Source: CAD feature listing. Evaluate the final solid. Frame: model axes, mm. A direction names the side the tool comes from. Coordinates: 2 decimals unless noted, no trailing zeros. Loops run counter-clockwise (first coordinate to the right, second up) from the corner with the lowest first, then second, coordinate; pieces in that order, holes last.
Item 1: Section query A-A, the plane x = 26. Return the cut outline in (y, z).
Item 2: Reachability of faces 1 (the flat face through (28, 0, 0)), 2 (the flat face through (28, -0.26, 0)), 3 (the flat face through (36, 0.013, 0)) from +Z, -Z, +X, -X, +Y, -Y: full face, straight path, thin tool, end or side. Return the list, or none.
Item 3: Line query: probe 1 along X at (y, z) = (-0.05, -8.25); probe 2 along Y at (x, z) = (36, -1.75); probe 3 along Z at (x, y) = (65.5, -0.1). Output: solid intervals per line, ascending.
Item 4: Section query D-D, the plane x = 10.5. Return the cut outline in (y, z).
Item 5: Pin query (flat end, axial travel): pin 1 Ø4 at (x, z) = (35.5, -1.5) entering from +Y. Return the tip coordinate at first contact, or that it passes through.
Item 6: Section query B-B, the plane y = -0.1. Return the cut outline in (x, z), then the cut area to 4 significant figures.
```python
from build123d import *

# Parameters (mm, degrees)
BOSS_EXTRUDE1_DEPTH      = 0.0001
BOSS_EXTRUDE1_DEPTH_BACK = 0.26
BOSS_EXTRUDE2_DEPTH      = 0.0126
BOSS_EXTRUDE3_DEPTH      = 0.0666


with BuildPart() as part:
    # Sketch1 → Boss-Extrude1 (new, two sides: drawn at the far end of the back side and taken through both)
    with BuildSketch(Plane(origin=(0, 0, 0), x_dir=(1, 0, 0), z_dir=(0, 1, 0)).offset(-BOSS_EXTRUDE1_DEPTH_BACK)):
        Polygon((0, -15), (30, -15), (30, -5), (74.5, -5), (74.5, 5), (30, 5), (30, 15), (0, 15), align=None)
    extrude(amount=BOSS_EXTRUDE1_DEPTH + BOSS_EXTRUDE1_DEPTH_BACK)

    # Sketch3 → Boss-Extrude2 (add)
    with BuildSketch(Plane(origin=(0, 0.0001, 0), x_dir=(1, 0, 0), z_dir=(0, 1, 0))):
        Polygon((30, 3.75), (30, 1.25), (35.5, 1.25), (35.5, -1.25), (30, -1.25), (30, -3.75), (38, -3.75), (38, 3.75), align=None)
    extrude(amount=BOSS_EXTRUDE2_DEPTH)

    # Sketch4 → Boss-Extrude3 (add)
    with BuildSketch(Plane(origin=(0, 0.0001, 0), x_dir=(1, 0, 0), z_dir=(0, 1, 0))):
        Polygon((4, 10.25), (4, 1.25), (30, 1.25), (30, 3.75), (20.627589053, 3.75), (20.627589053, 10.25), align=None)
        Polygon((30, -1.25), (4, -1.25), (4, -10.25), (20.627589053, -10.25), (20.627589053, -3.75), (30, -3.75), align=None)
    extrude(amount=BOSS_EXTRUDE3_DEPTH)


solid = part.part
```
Verdict:
1. outline: (-0.26, -15) - (0, -15) - (0, -3.75) - (0.07, -3.75) - (0.07, -1.25) - (0, -1.25) - (0, 1.25) - (0.07, 1.25) - (0.07, 3.75) - (0, 3.75) - (0, 15) - (-0.26, 15) - close
2. face 1: +Y
2. face 2: +Z, -Z, +X, -X, -Y
2. face 3: +Z, -Z, +X, +Y
3. probe 1: x = 0 to 30
3. probe 2: y = -0.26 to 0.01
3. probe 3: z = -5 to 5
4. outline: (-0.26, -15) - (0, -15) - (0, -10.25) - (0.07, -10.25) - (0.07, -1.25) - (0, -1.25) - (0, 1.25) - (0.07, 1.25) - (0.07, 10.25) - (0, 10.25) - (0, 15) - (-0.26, 15) - close
5. pin 1: stops at y = 0.01
6. outline: (0, -15) - (30, -15) - (30, -5) - (74.5, -5) - (74.5, 5) - (30, 5) - (30, 15) - (0, 15) - close
6. area: 1,345 mm2
